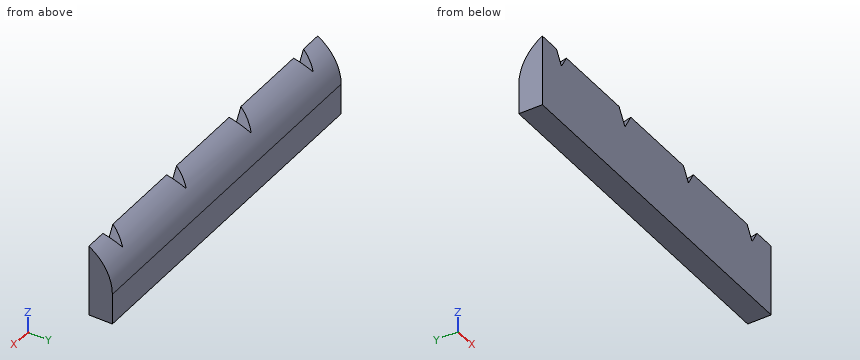
from build123d import *

# Parameters (mm, degrees)
F0_W        = 38.1
F0_H        = 2.54
F1_DEPTH    = 7.747
F3_T1_DEPTH = 60.0970452561
F4_DEPTH    = 25.4


# Not quite as in the source:
# - a fillet or chamfer that OpenCascade refuses, or shapes differently, is made with other operations: its cross-section is extruded or revolved along the edge and cut away or added


with BuildPart() as f1:
    # F0 (on Top) → F1 (new body)
    with BuildSketch(Plane.XY):
        with Locations((0, 1.27)):
            Rectangle(F0_W, F0_H)
    extrude(amount=F1_DEPTH)

    # F3: fillet of radius 5.08 on 1 edges, made by hand

    # F3_s2 → F3_t1 (cut)
    with BuildSketch(Plane.YZ.offset(-30.0485226281)):
        with BuildLine():
            ThreePointArc((2.54, 3.3475909488), (1.8594090512, 5.8875909488), (0, 7.747))
            Line((0, 7.747), (2.54, 7.747))
            Line((2.54, 7.747), (2.54, 3.3475909488))
        make_face()
    extrude(amount=F3_T1_DEPTH, mode=Mode.SUBTRACT)

    # F2 (on face) → F4 (cut)
    with BuildSketch(Plane.XZ):
        Polygon((-15.875, 6.3092954744), (-15.0449409051, 7.747), (-16.7050590949, 7.747), align=None)
        Polygon((-4.3191939367, 7.747), (-6.2726060633, 7.747), (-5.2959, 6.0552954744), align=None)
        Polygon((6.1005590949, 7.747), (4.4404409051, 7.747), (5.2705, 6.3092954744), align=None)
        Polygon((16.7050590949, 7.747), (15.0449409051, 7.747), (15.875, 6.3092954744), align=None)
    extrude(amount=-F4_DEPTH, mode=Mode.SUBTRACT)


solid = f1.part
Part model, mm, in its own coordinate system. Give positions to 0.01 mm unless a question says otherwise; leave off trailing zeros. Loops run counter-clockwise (first coordinate to the right, second up) from the corner with the lowest first, then second, coordinate; pieces in that order, holes last. Notation, with made-up numbers: (-35.5, -6.75) -> (22.5, -6.75) arc R21 ccw to (22.5, 4.25) -> close; hole circle Ø1 at (39.25, 47). An arc over 180 degrees is marked (long way). Write each question's results on one line, items separated by ' | '. Start each with the question number.
Q1. Band-saw the part on B-B on x = 1.5. List the corners of the cut face in (y, z), plus the area to 3 significant figures.
Q2. Wall check: L1, parallel to Y at x = 8.5, z = 3.5; L2, parallel to Z at x = -15, y = 0.35; L3, parallel to Z at x = 5.5, y = 0.8. Give the ranges that are in metal, low to high.
Q3. Band-saw the part on C-C on z = 4.75. List the corners of the cut face in (x, y), plus the area to 3 significant figures.
Results are:
1) outline: (0, 0) -> (2.54, 0) -> (2.54, 3.35) arc R5.08 ccw to (0, 7.75) -> close | area: 16.4 mm²
2) L1: y = 0 to 2.54 | L2: z = 0 to 7.53 | L3: z = 0 to 6.71
3) outline: (-19.05, 0) -> (19.05, 0) -> (19.05, 2.34) -> (-19.05, 2.34) -> close | area: 89.3 mm²
